Autodesk Inventor part; units mm, degrees
ref_plane "YZ Plane" through (0, 0, 0) normal (1, 0, 0) x (0, 1, 0)
ref_plane "XZ Plane" through (0, 0, 0) normal (0, 1, 0) x (-1, 0, 0)
ref_plane "XY Plane" through (0, 0, 0) normal (0, 0, 1) x (1, 0, 0)
sketch "Sketch1" plane through (0, 0, 0) normal (0, 1, 0) x (-1, 0, 0)
  line L0 (10.5834, 13.2197) -> (-45.9966, 13.2197)
  line L1 (-45.9966, 13.2197) -> (-45.9966, -11.7803)
  line L2 (-45.9966, -11.7803) -> (10.5834, -11.7803)
  line L3 (10.5834, -11.7803) -> (10.5834, 13.2197)
  circle A0 centre (5.5834, -7.8803) radius 1.55
  circle A1 centre (5.5834, 2.1197) radius 1.55
  circle A2 centre (-4.4166, 2.1197) radius 1.55
  circle A3 centre (-35.9966, 8.2197) radius 1.55
  circle A4 centre (-35.9966, -6.7803) radius 1.55
  point P0 (0, 0)
  dimension "d0" = 3.1
  dimension "d1" = 3.9
  dimension "d4" = 10
  dimension "d11" = 10
  dimension "d16" = 25
  dimension "d17" = 5
  dimension "d18" = 56.58
  dimension "d19" = 3.1
  dimension "d20" = 10
  dimension "d23" = 15
  dimension "d28" = 5
extrude "Extrusion1" add sketch "Sketch1" along normal mid plane 4
sketch "Sketch2" plane through (45.9966, 2, -11.7803) normal (0, 0, -1) x (-1, 0, 0)
  arc A0 (38.37, 0) -> (38.62, 0) centre (38.495, 0) ccw
  line L0 (0, 0) -> (56.58, 0)
  line L1 (56.58, -4) -> (56.58, 0)
  circle A1 centre (20, 0) radius 0.125
  line L2 (0, -4) -> (0, 0)
  point P0 (45.9966, -2)
  point P1 (56.58, -2)
  point P2 (20.125, 0)
  point P3 (19.875, 0)
  dimension "d31" = 0.25
  dimension "d34" = 18.085
  dimension "d35" = 0.25
  dimension "d36" = 20
extrude "Extrusion2" cut sketch "Sketch2" against normal up to surface (25 mm away) contours L0 A0 | A1 L0 picked at (20, -0.0736)
fillet "Fillet1" radius 0.1 4 edges at (7.6266, 2, 0.7197) (7.3766, 2, 0.7197) (26.1216, 2, 0.7197) (25.8716, 2, 0.7197)
fillet "Fillet2" radius 5 1 edges at (-10.5834, 0, 13.2197)
properties part number "GVS_Plate"
Source: CAD feature listing. Evaluate the final solid. Frame: model axes, mm. Round coordinates to 2 decimals unless told otherwise and drop trailing zeros. Order: outer loops, then holes, each group sorted by start corner. A loop starts at its lowest first (then second) coordinate and runs counter-clockwise, first axis right, second up. Notation, with made-up numbers: (89, 57) -> (136, 57) arc R23 ccw to (136, 67) -> close; hole circle Ø4 at (63, -14.5). An arc over 180 degrees is marked (long way). Use CSV: the item, a comma, the result in double quotes.
(1) Pull-direction query (Z, two-part tool) for faces 1 (the face through (34.52, -0.03, 7.75)), 2 (the face through (-10.583, 0, -2)), 3 (the face through (20, 0, 13.22)); classes: +Z half, -Z half, draft (parallel to the pull), parting line (faces both ways), or undercut.
Report:
face 1,"undercut"
face 2,"draft"
face 3,"+Z half"
(2) Ray query, L1, parallel to X at y = -0.9, z = 2.75; L2, parallel to X at y = -0.15, z = 2.5; L3, parallel to X at y = -0.8, z = -9. Return the intervals inside material, ascending.
Report:
L1,"-10.58 to -7, -4.17 to 3, 5.83 to 46"
L2,"-10.58 to -7.09, -4.08 to 2.91, 5.92 to 46"
L3,"-10.58 to -6.66, -4.51 to 46"
(3) First-contact query: pin 1 Ø3 at (x, z) = (-5.58, 2.12) entering from -Y. Flat tip, straight axial feed; report the tip coordinate or a pass-through.
Report:
pin 1,"through"
(4) Section A-A on y = -0.65. Return the cut outline in (x, z).
Report:
outline,"(-10.58, -11.78) -> (46, -11.78) -> (46, 13.22) -> (-5.58, 13.22) arc R5 ccw to (-10.58, 8.22) -> close; hole circle Ø3.1 at (-5.58, -7.88); hole circle Ø3.1 at (-5.58, 2.12); hole circle Ø3.1 at (4.42, 2.12); hole circle Ø3.1 at (36, -6.78); hole circle Ø3.1 at (36, 8.22)"
(5) Section B-B on z = 11. Return the cut outline in (x, y) (3 decimals), and give its area (3 significant figures).
Report:
outline,"(-9.739, -2) -> (45.997, -2) -> (45.997, 2) -> (26.198, 2) arc R0.1 ccw to (26.109, 1.944) arc R0.125 cw to (25.885, 1.944) arc R0.1 ccw to (25.795, 2) -> (7.703, 2) arc R0.1 ccw to (7.614, 1.944) arc R0.125 cw to (7.39, 1.944) arc R0.1 ccw to (7.3, 2) -> (-9.739, 2) -> close"
area,"223 mm^2"
